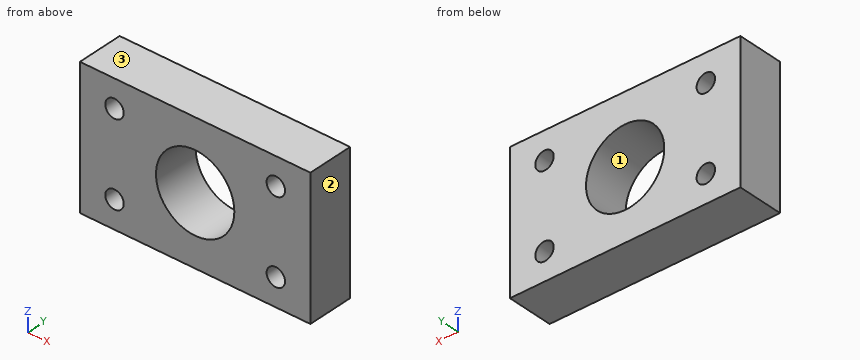
from build123d import *

# Parameters (mm, degrees)
SKETCH1_W           = 50
SKETCH1_H           = 30
SKETCH1_R           = 8.5
SKETCH1_R_2         = 2
BOSS_EXTRUDE1_DEPTH = 10


with BuildPart() as part:
    # Sketch1 → Boss-Extrude1 (new body)
    with BuildSketch(Plane(origin=(0, 0, 0), x_dir=(1, 0, 0), z_dir=(0, 1, 0))):
        Rectangle(SKETCH1_W, SKETCH1_H)
        Circle(SKETCH1_R, mode=Mode.SUBTRACT)
        with Locations((-17.5, 9)):
            Circle(SKETCH1_R_2, mode=Mode.SUBTRACT)
        with Locations((17.5, 9)):
            Circle(SKETCH1_R_2, mode=Mode.SUBTRACT)
        with Locations((17.5, -9)):
            Circle(SKETCH1_R_2, mode=Mode.SUBTRACT)
        with Locations((-17.5, -9)):
            Circle(SKETCH1_R_2, mode=Mode.SUBTRACT)
    extrude(amount=BOSS_EXTRUDE1_DEPTH)


solid = part.part
Can you work these out from the model? Positions are in its coordinate system, mm. Face numbers are marked on the shaded views. Coordinates: 2 decimals unless noted, no trailing zeros. Order: outer loops, then holes, each group sorted by start corner. A loop starts at its lowest first (then second) coordinate and runs counter-clockwise, first axis right, second up. Notation, with made-up numbers: (-30.75, 20.25) - (6.25, 20.25) arc R24 cw to (6.25, 30.25) - close; hole circle Ø1 at (44, 75.5). An arc over 180 degrees is marked (long way). Answer as a JSON object with one key per item and string values. Group by question number.
Q1. Imagine slicing it at A-A (x = 17.5). Please give me the cut outline in (y, z).
Q2. Imagine slicing it at B-B (z = 9). Please give me the cut outline in (x, y).
Q3. We'd pull the mould along Z, two halves only. Please class the marked faces 1, 2 and 3: +Z half, -Z half, draft (parallel to the pull), parting line (faces both ways), or undercut.
Q4. Imagine slicing it at C-C (x = 0). Please give me the cut outline in (y, z).
Q5. Will these pins go through, and if not, where does the flat tip stop? P1, Ø3, axis at x = 17.5, z = -9, coming from the +Y side; P2, Ø6.5, axis at x = -17.5, z = 9, coming from the -Y side.
Q6. I need wall thicknesses on line 1 (Z direction, x = -17.5, y = 4.5); line 2 (X direction, y = 6, z = 9); line 3 (X direction, y = 7, z = 0). Which ranges of each line are inside material? Lowest first, please. Write a range as from..to.
Q7. Imagine slicing it at D-D (y = 8). Please give me the cut outline in (x, z).
Determined:
{
 "1": {"outline": "(0, -15) - (10, -15) - (10, -11) - (0, -11) - close; (0, -7) - (10, -7) - (10, 7) - (0, 7) - close; (0, 11) - (10, 11) - (10, 15) - (0, 15) - close"},
 "2": {"outline": "(-25, 0) - (-19.5, 0) - (-19.5, 10) - (-25, 10) - close; (-15.5, 0) - (15.5, 0) - (15.5, 10) - (-15.5, 10) - close; (19.5, 0) - (25, 0) - (25, 10) - (19.5, 10) - close"},
 "3": {"face 1": "undercut", "face 2": "draft", "face 3": "+Z half"},
 "4": {"outline": "(0, -15) - (10, -15) - (10, -8.5) - (0, -8.5) - close; (0, 8.5) - (10, 8.5) - (10, 15) - (0, 15) - close"},
 "5": {"P1": "passes through", "P2": "stops at y = 0"},
 "6": {"line 1": "z = -15..-11, -7..7, 11..15", "line 2": "x = -25..-19.5, -15.5..15.5, 19.5..25", "line 3": "x = -25..-8.5, 8.5..25"},
 "7": {"outline": "(-25, -15) - (25, -15) - (25, 15) - (-25, 15) - close; hole circle Ø4 at (-17.5, -9); hole circle Ø4 at (-17.5, 9); hole circle Ø17 at (0, 0); hole circle Ø4 at (17.5, -9); hole circle Ø4 at (17.5, 9)"}
}
